from build123d import *

# Parameters (mm, degrees)
SKETCH1_R           = 2.54
SKETCH1_R_2         = 2.4892
BOSS_EXTRUDE1_DEPTH = 2.286
FILLET1_R           = 6.35


with BuildPart() as part:
    # Sketch1 → Boss-Extrude1 (new body)
    with BuildSketch(Plane(origin=(0, 0, -219.608471563), x_dir=(-1, 0, 0), z_dir=(0, 0, -1))):
        Polygon((77.53656774, 159.000825673), (77.53656774, 108.200825673), (-17.71343226, 108.200825673), (-17.71343226, 222.500825674), (33.08656774, 222.500825674), (33.08656774, 159.000825673), align=None)
        with Locations((44.553419861, 120.900826428)):
            Circle(SKETCH1_R, mode=Mode.SUBTRACT)
        with Locations((57.257798242, 133.600825673)):
            Circle(SKETCH1_R, mode=Mode.SUBTRACT)
        with Locations((69.957798242, 146.300825673)):
            Circle(SKETCH1_R, mode=Mode.SUBTRACT)
        with Locations((69.957798242, 133.600825673)):
            Circle(SKETCH1_R, mode=Mode.SUBTRACT)
        with Locations((69.957798242, 120.900825673)):
            Circle(SKETCH1_R, mode=Mode.SUBTRACT)
        with Locations((57.253419861, 120.900826428)):
            Circle(SKETCH1_R, mode=Mode.SUBTRACT)
        with Locations((20.38656774, 165.350825674)):
            Circle(SKETCH1_R_2, mode=Mode.SUBTRACT)
        with Locations((-6.242201758, 146.300824919)):
            Circle(SKETCH1_R, mode=Mode.SUBTRACT)
        with Locations((-6.246580139, 133.600825673)):
            Circle(SKETCH1_R, mode=Mode.SUBTRACT)
        with Locations((6.457798242, 146.300825673)):
            Circle(SKETCH1_R, mode=Mode.SUBTRACT)
        with Locations((6.453419861, 133.600826428)):
            Circle(SKETCH1_R, mode=Mode.SUBTRACT)
        with Locations((19.157798242, 146.300825673)):
            Circle(SKETCH1_R, mode=Mode.SUBTRACT)
        with Locations((-6.246580139, 120.900825673)):
            Circle(SKETCH1_R, mode=Mode.SUBTRACT)
        with Locations((6.453419861, 120.900826428)):
            Circle(SKETCH1_R, mode=Mode.SUBTRACT)
        with Locations((19.153419861, 120.900826428)):
            Circle(SKETCH1_R, mode=Mode.SUBTRACT)
        with Locations((19.157798242, 133.600825673)):
            Circle(SKETCH1_R, mode=Mode.SUBTRACT)
        with Locations((31.857798242, 133.600825673)):
            Circle(SKETCH1_R, mode=Mode.SUBTRACT)
        with Locations((44.557798242, 133.600825673)):
            Circle(SKETCH1_R, mode=Mode.SUBTRACT)
        with Locations((31.857798242, 146.300825673)):
            Circle(SKETCH1_R, mode=Mode.SUBTRACT)
        with Locations((44.557798242, 146.300825673)):
            Circle(SKETCH1_R, mode=Mode.SUBTRACT)
        with Locations((57.257798242, 146.300825673)):
            Circle(SKETCH1_R, mode=Mode.SUBTRACT)
        with Locations((31.853419861, 120.900826428)):
            Circle(SKETCH1_R, mode=Mode.SUBTRACT)
        with Locations((-5.01343226, 216.150825674)):
            Circle(SKETCH1_R_2, mode=Mode.SUBTRACT)
        with Locations((7.68656774, 216.150825674)):
            Circle(SKETCH1_R_2, mode=Mode.SUBTRACT)
        with Locations((20.38656774, 216.150825674)):
            Circle(SKETCH1_R_2, mode=Mode.SUBTRACT)
        with Locations((-5.01343226, 203.450825674)):
            Circle(SKETCH1_R_2, mode=Mode.SUBTRACT)
        with Locations((7.68656774, 203.450825674)):
            Circle(SKETCH1_R_2, mode=Mode.SUBTRACT)
        with Locations((20.38656774, 203.450825674)):
            Circle(SKETCH1_R_2, mode=Mode.SUBTRACT)
        with Locations((-5.01343226, 190.750825674)):
            Circle(SKETCH1_R_2, mode=Mode.SUBTRACT)
        with Locations((7.68656774, 190.750825674)):
            Circle(SKETCH1_R_2, mode=Mode.SUBTRACT)
        with Locations((20.38656774, 190.750825674)):
            Circle(SKETCH1_R_2, mode=Mode.SUBTRACT)
        with Locations((-5.01343226, 178.050825674)):
            Circle(SKETCH1_R_2, mode=Mode.SUBTRACT)
        with Locations((7.68656774, 178.050825674)):
            Circle(SKETCH1_R_2, mode=Mode.SUBTRACT)
        with Locations((20.38656774, 178.050825674)):
            Circle(SKETCH1_R_2, mode=Mode.SUBTRACT)
        with Locations((-5.01343226, 165.350825674)):
            Circle(SKETCH1_R_2, mode=Mode.SUBTRACT)
        with Locations((7.68656774, 165.350825674)):
            Circle(SKETCH1_R_2, mode=Mode.SUBTRACT)
    extrude(amount=BOSS_EXTRUDE1_DEPTH)

    # Fillet1
    fillet1_edges = [part.edges().sort_by_distance(p)[0] for p in [
        (17.71343226, 108.200825673, -220.751471563),
        (17.71343226, 222.500825674, -220.751471563),
        (-33.08656774, 222.500825674, -220.751471563),
        (-33.08656774, 159.000825673, -220.751471563),
        (-77.53656774, 159.000825673, -220.751471563),
        (-77.53656774, 108.200825673, -220.751471563),
    ]]
    fillet(fillet1_edges, radius=FILLET1_R)


solid = part.part
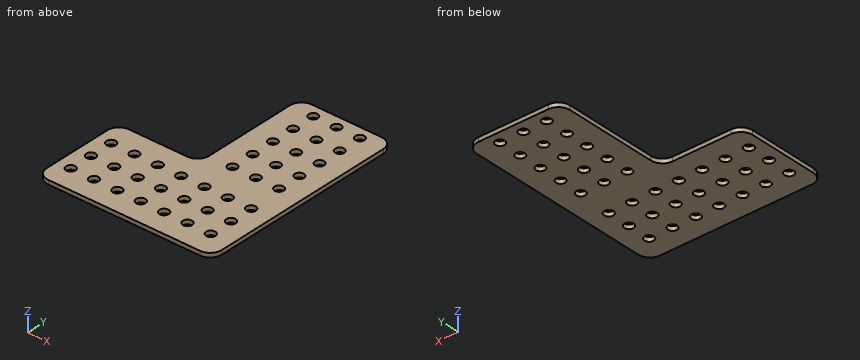
Check sheet for the modelled part. Datum: model origin and axes. Units: mm. Round coordinates to 2 decimals unless told otherwise and drop trailing zeros. Loops run counter-clockwise (first coordinate to the right, second up) from the corner with the lowest first, then second, coordinate; pieces in that order, holes last. Notation, with made-up numbers: (-38.5, 28.25) - (-27.5, 28.25) arc R34 ccw to (-27.5, 60.25) - close; hole circle Ø4 at (-0.75, 54). An arc over 180 degrees is marked (long way). Answer as CSV lines item,"result". Start each with the question number.
Item 1: Depth check by flat-ended pin: P1, Ø6.5, axis at x = -69.96, y = 133.6, coming from the +Z side; P2, Ø4.5, axis at x = -19.15, y = 120.9, coming from the +Z side. Enter the tip coordinate at first touch or a pass-through.
Item 2: Section check B-B (x = -61). Record the boundary of the cut face in (y, z), and give its area (3 significant figures).
Item 3: Scan lines: line 1 (X direction, y = 203, z = -220.8); line 2 (Y direction, x = -57, z = -221.45); line 3 (X direction, y = 214.5, z = -220.85). Record each from-to range of solid material in increasing order. Write a range as [from, to].
Item 4: Section check C-C (x = -37). Record the boundary of the cut face in (y, z), and give its area (3 significant figures).
Item 5: Section check A-A (z = -220.8). Count the separate pieces of the cut face and the enclosed holes in it, and give its area (3 significant figures).
Report:
1,P1,"stops at z = -219.61"
1,P2,"passes through"
2,outline,"(108.2, -221.89) - (159, -221.89) - (159, -219.61) - (108.2, -219.61) - close"
2,area,"116 mm2"
3,line 1,"x = [-33.09, -22.83], [-17.94, -10.13], [-5.24, 2.57], [7.46, 17.71]"
3,line 2,"y = [108.2, 118.37], [123.43, 131.07], [136.13, 143.77], [148.83, 159]"
3,line 3,"x = [-33.09, -22.25], [-18.52, -9.55], [-5.82, 3.15], [6.88, 17.71]"
4,outline,"(108.2, -221.89) - (159.49, -221.89) - (159.49, -219.61) - (108.2, -219.61) - close"
4,area,"117 mm2"
5,separate pieces,"1"
5,enclosed holes,"36"
5,area,"7,310 mm2"
